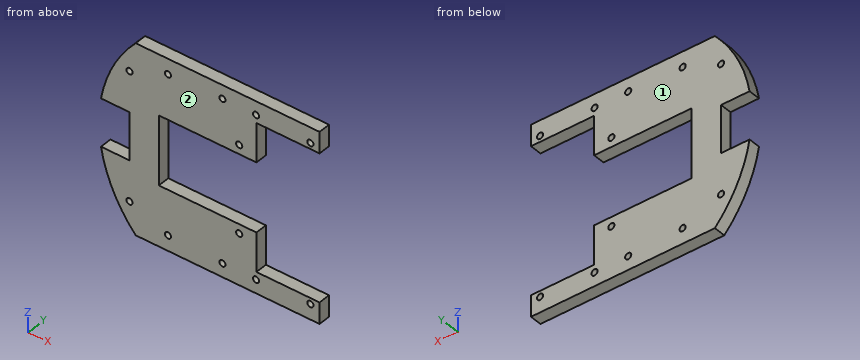
```python
from build123d import *

# Parameters (mm, degrees)
SKETCH1_R           = 1.651
BOSS_EXTRUDE1_DEPTH = 6.35


with BuildPart() as part:
    # Sketch1 → Boss-Extrude1 (new body)
    with BuildSketch(Plane(origin=(0, 0, 0), x_dir=(1, 0, 0), z_dir=(0, 1, 0))):
        with BuildLine():
            Line((33.776652136, 7.168881649), (0, 7.168881649))
            Line((0, 7.168881649), (0, 44.052727236))
            Line((0, 44.052727236), (33.776652136, 44.052727236))
            Line((33.776652136, 44.052727236), (52.191652136, 44.052727236))
            Line((52.191652136, 44.052727236), (52.191652136, 64.853804442))
            Line((52.191652136, 64.853804442), (85.968304273, 64.853804442))
            Line((85.968304273, 64.853804442), (85.968304273, 76.214266248))
            Line((85.968304273, 76.214266248), (0, 76.214266248))
            Line((0, 76.214266248), (-12.371874213, 76.214266248))
            ThreePointArc((-12.371874213, 76.214266248), (-24.373410945, 58.595023332), (-30.932760678, 38.310804442))
            Line((-30.932760678, 38.310804442), (-15.692760678, 38.310804442))
            Line((-15.692760678, 38.310804442), (-15.692760678, 12.910804442))
            Line((-15.692760678, 12.910804442), (-30.932760678, 12.910804442))
            ThreePointArc((-30.932760678, 12.910804442), (-24.373410945, -7.373414447), (-12.371874213, -24.992657364))
            Line((-12.371874213, -24.992657364), (0, -24.992657364))
            Line((0, -24.992657364), (85.968304273, -24.992657364))
            Line((85.968304273, -24.992657364), (85.968304273, -13.632195558))
            Line((85.968304273, -13.632195558), (52.191652136, -13.632195558))
            Line((52.191652136, -13.632195558), (52.191652136, 7.168881649))
            Line((52.191652136, 7.168881649), (33.776652136, 7.168881649))
        make_face()
        with Locations(Location((4.884152136, -16.807195558, 0), (0, 0, 270))):
            Circle(SKETCH1_R, mode=Mode.SUBTRACT)
        with Locations(Location((81.084152136, -16.807195558, 0), (0, 0, 270))):
            Circle(SKETCH1_R, mode=Mode.SUBTRACT)
        with Locations(Location((42.984152136, 2.242804442, 0), (0, 0, 270))):
            Circle(SKETCH1_R, mode=Mode.SUBTRACT)
        with Locations(Location((33.983402136, -17.742657364, 0), (0, 0, 270))):
            Circle(SKETCH1_R, mode=Mode.SUBTRACT)
        with Locations(Location((51.983402136, -17.742657364, 0), (0, 0, 270))):
            Circle(SKETCH1_R, mode=Mode.SUBTRACT)
        with Locations(Location((51.983402136, 68.964266248, 0), (0, 0, 90))):
            Circle(SKETCH1_R, mode=Mode.SUBTRACT)
        with Locations(Location((33.983402136, 68.964266248, 0), (0, 0, 90))):
            Circle(SKETCH1_R, mode=Mode.SUBTRACT)
        with Locations(Location((42.984152136, 48.978804442, 0), (0, 0, 90))):
            Circle(SKETCH1_R, mode=Mode.SUBTRACT)
        with Locations(Location((81.084152136, 68.028804442, 0), (0, 0, 90))):
            Circle(SKETCH1_R, mode=Mode.SUBTRACT)
        with Locations(Location((4.884152136, 68.028804442, 0), (0, 0, 90))):
            Circle(SKETCH1_R, mode=Mode.SUBTRACT)
        with Locations(Location((-15.692760678, 59.900804442, 0), (0, 0, 270))):
            Circle(SKETCH1_R, mode=Mode.SUBTRACT)
        with Locations(Location((-15.692760678, -8.679195558, 0), (0, 0, 270))):
            Circle(SKETCH1_R, mode=Mode.SUBTRACT)
    extrude(amount=BOSS_EXTRUDE1_DEPTH)


solid = part.part
```
Verification items for the finished model (mm, model axes). Face numbers are marked on the shaded views. Round coordinates to 2 decimals unless told otherwise and drop trailing zeros. Write each loop counter-clockwise with the first axis right and the second up, starting at its lowest first coordinate (ties: lowest second). Pieces come first, ordered by that corner, then holes. Notation, with made-up numbers: (-3, -33.75) -> (38, -33.75) arc R19 ccw to (38, -16.75) -> close; hole circle Ø2 at (4, 81.25). An arc over 180 degrees is marked (long way). Write each question's results on one line, items separated by ' | '.
Q1. Sectioned sample at D-D, the plane z = 3.5. Record the boundary of the cut face in (x, y), and give its area (3 significant figures).
Derived:
outline: (-26.14, 0) -> (52.19, 0) -> (52.19, 6.35) -> (-26.14, 6.35) -> close | area: 497 mm²
Q2. Thickness scan on probe 1 along Z at (x, y) = (37, 4.75); probe 2 along Z at (x, y) = (78, 4.5); probe 3 along Z at (x, y) = (44, 3.75). Record the ranges inside material, lowest first.
Derived:
probe 1: z = -76.21 to -44.05, -7.17 to 24.99 | probe 2: z = -76.21 to -64.85, 13.63 to 24.99 | probe 3: z = -76.21 to -50.28, -47.68 to -44.05, -7.17 to -3.54, -0.94 to 24.99
Q3. Sectioned sample at B-B, the plane y = 3.25. Give the number of separate pieces and of enclosed holes in the cut face, and give its area (3 significant figures).
Derived:
separate pieces: 1 | enclosed holes: 12 | area: 6,230 mm²
Q4. Sectioned sample at A-A, the plane x = 29. Record the boundary of the cut face in (y, z), and give its area (3 significant figures).
Derived:
outline: (0, -76.21) -> (6.35, -76.21) -> (6.35, -44.05) -> (0, -44.05) -> close; (0, -7.17) -> (6.35, -7.17) -> (6.35, 24.99) -> (0, 24.99) -> close | area: 408 mm²
Q5. Draft check along Y on the marked faces 1 and 2. Enter one of: released by +Y, released by -Y, zero draft, split by the parting line, or undercut.
Derived:
face 1: released by +Y | face 2: released by -Y
Q6. Go/stop test with flat-tipped pins: pin 1 Ø3 at (y, z) = (4, -9.5) entering from +X; pin 2 Ø2 at (x, z) = (81.08, -68.03) entering from +Y; pin 3 Ø1.9 at (x, y) = (-25, 3.5) entering from -Z; pin 4 Ø3 at (x, y) = (-26, 4) entering from +Z. Record where each tip stops, or that it passes through.
Derived:
pin 1: stops at x = 0 | pin 2: passes through | pin 3: stops at z = -59.25 | pin 4: stops at z = 7.11
Q7. Sectioned sample at C-C, the plane z = -33.5. Record the boundary of the cut face in (x, y).
Derived:
outline: (-15.69, 0) -> (0, 0) -> (0, 6.35) -> (-15.69, 6.35) -> close
